The drawing under review shows one solid part. Ordinate dimensions are in mm from its lowest x, y, z. Round coordinates to 2 decimals unless told otherwise and drop trailing zeros. Write each loop counter-clockwise with the first axis right and the second up, starting at its lowest first coordinate (ties: lowest second). Pieces come first, ordered by that corner, then holes. Notation, with made-up numbers: (-22.75, 56.5) -> (26.25, 56.5) arc R13 cw to (26.25, 78.5) -> close; hole circle Ø6 at (-16.75, -34). An arc over 180 degrees is marked (long way). Use CSV: the item, a comma, the result in double quotes. Start each with the question number.
1) Take a section at A-A, the plane x = 65. Give the boundary of the cut face in (y, z).
2) Take a section at C-C, the plane x = 83. Give the boundary of the cut face in (y, z).
3) Mouldability with a two-part tool opening along Y and no side actions: class the marked faces 1, 2 and 3 as released by +Y, released by -Y, zero draft, split by the parting line, or undercut.
4) For pin 1 Ø5 at (y, z) = (84, 21) entering from -X; pin 2 Ø8 at (x, z) = (55.5, 15.5) entering from -Y; pin 3 Ø4.5 at (x, y) = (65, 2.5) entering from +Z; pin 4 Ø1.5 at (x, z) = (56.5, 37) entering from -Y, all flat-tipped, find the tip position at first contact; note any pin that passes through.
5) Take a section at D-D, the plane z = 34. Give the boundary of the cut face in (x, y), then the cut area to 3 significant figures.
6) Wall thickness on probe 1 along Y at (x, z) = (65, 48.4); probe 2 along Y at (x, z) = (65, 26); probe 3 along Z at (x, y) = (15.5, 105): over which ranges is each line inside the solid? List them lowest first. Write a range as [from, to].
7) Take a section at B-B, the plane y = 65. Give the boundary of the cut face in (x, z), then the cut area to 3 significant figures.
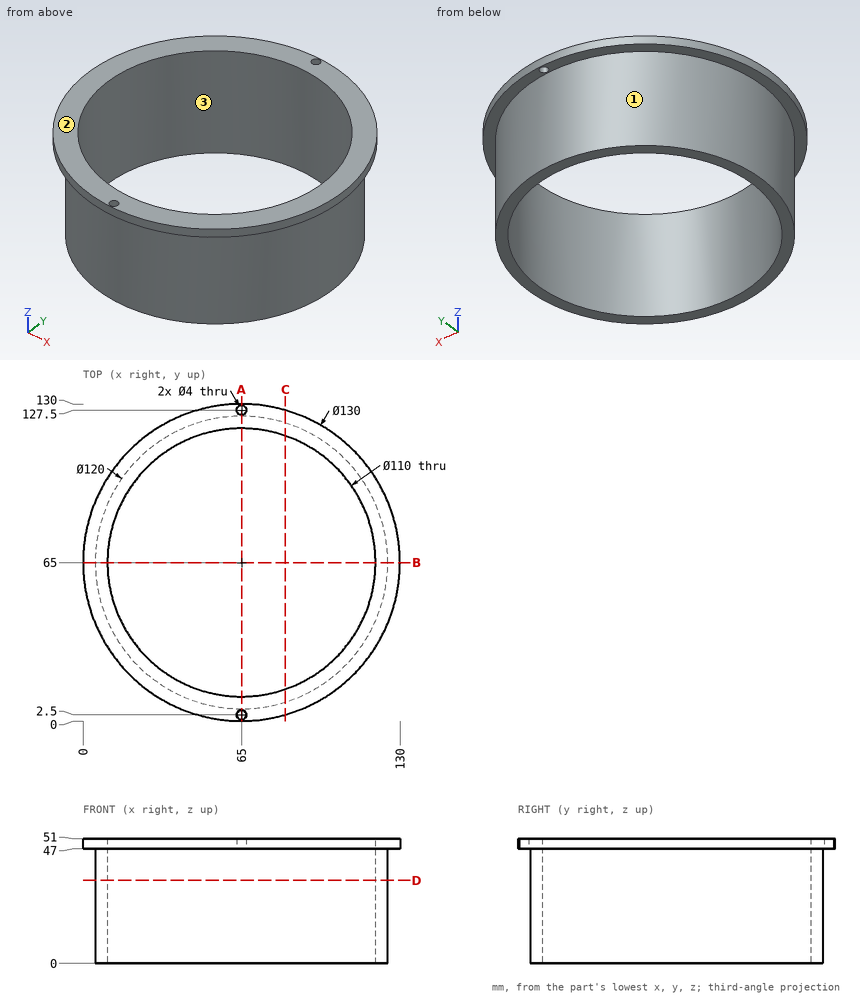
Values found:
1,outline,"(0, 47) -> (0.5, 47) -> (0.5, 51) -> (0, 51) -> close; (4.5, 47) -> (5, 47) -> (5, 0) -> (10, 0) -> (10, 51) -> (4.5, 51) -> close; (120, 0) -> (125, 0) -> (125, 47) -> (125.5, 47) -> (125.5, 51) -> (120, 51) -> close; (129.5, 47) -> (130, 47) -> (130, 51) -> (129.5, 51) -> close"
2,outline,"(2.54, 47) -> (7.76, 47) -> (7.76, 0) -> (13.03, 0) -> (13.03, 51) -> (2.54, 51) -> close; (116.97, 0) -> (122.24, 0) -> (122.24, 47) -> (127.46, 47) -> (127.46, 51) -> (116.97, 51) -> close"
3,face 1,"split by the parting line"
3,face 2,"zero draft"
3,face 3,"undercut"
4,pin 1,"x = 7.31"
4,pin 2,"y = 5.25"
4,pin 3,"z = 51"
4,pin 4,"y = 5.5"
5,outline,"circle Ø120 at (65, 65); hole circle Ø110 at (65, 65)"
5,area,"1,810 mm²"
6,probe 1,"[0, 0.5], [4.5, 10], [120, 125.5], [129.5, 130]"
6,probe 2,"[5, 10], [120, 125]"
6,probe 3,"[47, 51]"
7,outline,"(0, 47) -> (5, 47) -> (5, 0) -> (10, 0) -> (10, 51) -> (0, 51) -> close; (120, 0) -> (125, 0) -> (125, 47) -> (130, 47) -> (130, 51) -> (120, 51) -> close"
7,area,"550 mm²"
